from build123d import *

# Parameters (mm, degrees)
SKETCH1_W           = 35
SKETCH1_H           = 100
BOSS_EXTRUDE1_DEPTH = 3.175
SKETCH2_R           = 1.5
SKETCH2_W           = 6.5
SKETCH2_H           = 42.5
CUT_EXTRUDE1_DEPTH  = 4.175
FILLET1_R           = 3
CHAMFER1_SIZE       = 3
CHAMFER1_SIZE2      = 1.732050808
SKETCH3_R           = 1
CUT_EXTRUDE2_DEPTH  = 4.175
SKETCH4_R           = 1.25
CUT_EXTRUDE3_DEPTH  = 4.175


with BuildPart() as part:
    # Sketch1 → Boss-Extrude1 (new body)
    with BuildSketch(Plane.XY):
        Rectangle(SKETCH1_W, SKETCH1_H)
    extrude(amount=BOSS_EXTRUDE1_DEPTH)

    # Sketch2 → Cut-Extrude1 (cut, through all)
    with BuildSketch(Plane.XY.offset(3.175)):
        with Locations((-7.5, 39)):
            Circle(SKETCH2_R)
        with Locations((-7.5, 11)):
            Circle(SKETCH2_R)
        with Locations((7.5, 11)):
            Circle(SKETCH2_R)
        with Locations((7.5, 39)):
            Circle(SKETCH2_R)
        with Locations((-14.25, 28.75)):
            Rectangle(SKETCH2_W, SKETCH2_H)
        with Locations((14.25, 28.75)):
            Rectangle(SKETCH2_W, SKETCH2_H)
    extrude(amount=-CUT_EXTRUDE1_DEPTH, mode=Mode.SUBTRACT)

    # Fillet1
    fillet1_edges = [part.edges().sort_by_distance(p)[0] for p in [
        (-17.5, 7.5, 1.5875),
        (-11, 50, 1.5875),
        (-11, 7.5, 1.5875),
        (11, 7.5, 1.5875),
        (11, 50, 1.5875),
        (17.5, 7.5, 1.5875),
    ]]
    fillet(fillet1_edges, radius=FILLET1_R)

    # Chamfer1
    chamfer1_edges = [part.edges().sort_by_distance(p)[0] for p in [
        (0, -50, 0),
    ]]
    chamfer1_side = [part.faces().sort_by_distance(p)[0] for p in [
        (0, -5.754552851, 0),
    ]]
    chamfer(chamfer1_edges, length=CHAMFER1_SIZE, length2=CHAMFER1_SIZE2, reference=chamfer1_side[0])

    # Sketch3 → Cut-Extrude2 (cut, through all)
    with BuildSketch(Plane.XY.offset(3.175)):
        with Locations((-4.75, 46)):
            Circle(SKETCH3_R)
        with Locations((4.75, 46)):
            Circle(SKETCH3_R)
    extrude(amount=-CUT_EXTRUDE2_DEPTH, mode=Mode.SUBTRACT)

    # Sketch4 → Cut-Extrude3 (cut, through all)
    with BuildSketch(Plane.XY.offset(3.175)):
        with Locations((-12.5, -45)):
            Circle(SKETCH4_R)
        with Locations((12.5, -45)):
            Circle(SKETCH4_R)
        with Locations((-12.5, -20)):
            Circle(SKETCH4_R)
        with Locations((12.5, -20)):
            Circle(SKETCH4_R)
        with Locations((0, -45)):
            Circle(SKETCH4_R)
        with Locations((0, -20)):
            Circle(SKETCH4_R)
    extrude(amount=-CUT_EXTRUDE3_DEPTH, mode=Mode.SUBTRACT)


solid = part.part
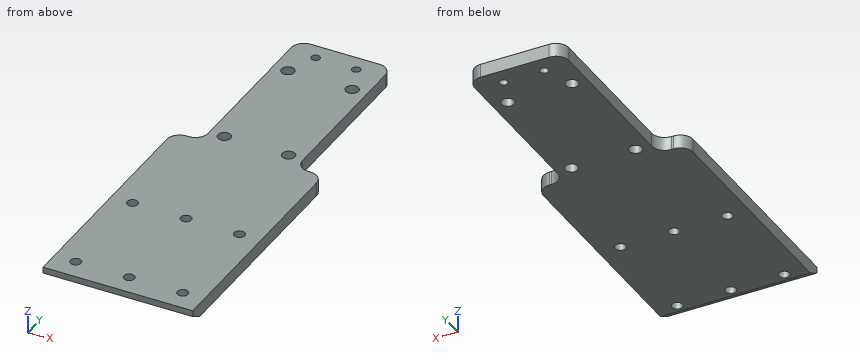
Model file for the job. Use its own axes, mm. Coordinates: 2 decimals unless noted, no trailing zeros. Write each loop counter-clockwise with the first axis right and the second up, starting at its lowest first coordinate (ties: lowest second). Pieces come first, ordered by that corner, then holes. Notation, with made-up numbers: (74.25, -23) -> (120.25, -23) arc R18 ccw to (120.25, -19) -> close; hole circle Ø11 at (-13.5, 59.25). An arc over 180 degrees is marked (long way). One line per item, written item: value. Start each with the question number.
1) Slice it at C-C on z = 2.4. Count the separate pieces of the cut face and the enclosed holes in it, then the cut area to 3 significant figures.
2) Probe probe 1 along Y at (x, z) = (7.5, 2.1); probe 2 along Y at (x, z) = (8, 1.8); probe 3 along X at (y, z) = (10, 1.95). List the from-to ranges inside material, lowest first.
3) Flat gauge pins, fed straight in: pin 1 Ø2.5 at (x, y) = (-7.5, 39) entering from -Z; pin 2 Ø1 at (y, z) = (16, 1) entering from +X; pin 3 Ø0.6 at (x, z) = (-14.5, 2) entering from +Y; pin 4 Ø1.6 at (y, z) = (25, 1.5) entering from -X. Where does each tip first touch, or does it go through?
4) Slice it at D-D on x = 12.5. Write the cut outline in (y, z) (3 decimals), then the cut area to 3 significant figures.
5) Slice it at B-B on y = 39. Write the cut outline in (x, z) (3 decimals).
6) Slice it at A-A on x = -4.75. Write the cut outline in (y, z) (3 decimals), then the cut area to 3 significant figures.
Answers follow:
1. separate pieces: 1
1. enclosed holes: 12
1. area: 2,880 mm2
2. probe 1: -50 to 9.5, 12.5 to 37.5, 40.5 to 50
2. probe 2: -50 to 9.59, 12.41 to 37.59, 40.41 to 50
2. probe 3: -11.04 to -8.62, -6.38 to 6.38, 8.62 to 11.04
3. pin 1: through
3. pin 2: x = 11
3. pin 3: y = 7.5
3. pin 4: x = -11
4. outline: (-50, 1.732) -> (-47, 0) -> (-46.25, 0) -> (-46.25, 3.175) -> (-50, 3.175) -> close; (-43.75, 0) -> (-21.25, 0) -> (-21.25, 3.175) -> (-43.75, 3.175) -> close; (-18.75, 0) -> (7.902, 0) -> (7.902, 3.175) -> (-18.75, 3.175) -> close
4. area: 165 mm2
5. outline: (-11, 0) -> (-9, 0) -> (-9, 3.175) -> (-11, 3.175) -> close; (-6, 0) -> (6, 0) -> (6, 3.175) -> (-6, 3.175) -> close; (9, 0) -> (11, 0) -> (11, 3.175) -> (9, 3.175) -> close
6. outline: (-50, 1.732) -> (-47, 0) -> (45, 0) -> (45, 3.175) -> (-50, 3.175) -> close; (47, 0) -> (50, 0) -> (50, 3.175) -> (47, 3.175) -> close
6. area: 309 mm2
